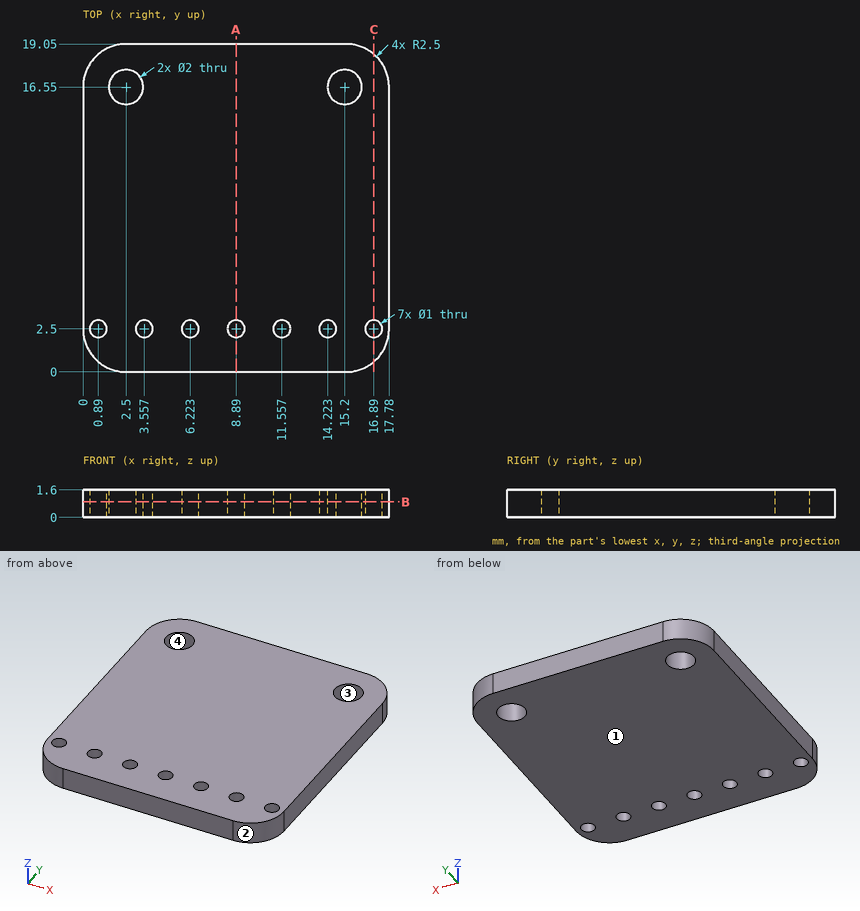
Answer from the drawing. Dimensions are ordinates in mm from the lowest x, y and z of the part. Coordinates: 2 decimals unless noted, no trailing zeros. Loops run counter-clockwise (first coordinate to the right, second up) from the corner with the lowest first, then second, coordinate; pieces in that order, holes last.
Q1. The part is cut by section A-A on x = 8.89. Write down the section's boundary in (y, z).
Q2. The mould has two halves that part along X. Classify the marked faces 1, 2, 3 and 4: +X half, -X half, draft (parallel to the pull), parting line (faces both ways), or undercut.
Q3. This flat-tipped pin is pushed along its axis until it touches: pin 1 Ø4 at (x, y) = (9, 2.5) entering from +Z. Where does it stop, or does it pass through?
Q4. Consider probe 1 along X at (y, z) = (16.5, 0.7); probe 2 along Y at (x, z) = (15.25, 0.45); probe 3 along Y at (x, z) = (16.75, 0.2). Determine where each line is inside the solid, lowest interval first.
Q5. The part is cut by section C-C on x = 16.89. Write down the section's boundary in (y, z).
Q6. The part is cut by section B-B on z = 0.9. Give the number of separate pieces and of enclosed holes in the cut face.
Results below:
1. outline: (0, 0) - (2, 0) - (2, 1.6) - (0, 1.6) - close; (3, 0) - (19.05, 0) - (19.05, 1.6) - (3, 1.6) - close
2. face 1: draft
2. face 2: +X half
2. face 3: undercut
2. face 4: undercut
3. pin 1: stops at z = 1.6
4. probe 1: x = 0 to 1.5, 3.5 to 14.2, 16.2 to 17.78
4. probe 2: y = 0 to 15.55, 17.55 to 19.05
4. probe 3: y = 0.48 to 2.02, 2.98 to 18.57
5. outline: (0.59, 0) - (2, 0) - (2, 1.6) - (0.59, 1.6) - close; (3, 0) - (18.46, 0) - (18.46, 1.6) - (3, 1.6) - close
6. separate pieces: 1
6. enclosed holes: 9
